Could you check a few things on this drawing? It's one solid part, dimensions in mm from its lowest x, y, z. Give positions to 0.01 mm unless a question says otherwise; leave off trailing zeros. Loops run counter-clockwise (first coordinate to the right, second up) from the corner with the lowest first, then second, coordinate; pieces in that order, holes last.
1. I need wall thicknesses on line 1 along X through (y, z) = (0.45, 4.45); line 2 along Y through (x, z) = (2.6, 4.45); line 3 along Z through (x, y) = (1.4, 1.5). Which ranges of each line are inside material? Lowest first, please.
2. Thinking about a two-plate mould opening in Z: for the marked faces 1, 2 and 3, which applies, +Z half, -Z half, draft (parallel to the pull), parting line (faces both ways), or undercut?
3. Imagine slicing it at D-D (z = 4.25). Count the separate pieces of the cut face and the enclosed holes in it.
4. Imagine slicing it at A-A (y = 1.5). List the corners of the cut face in (x, z) for me.
5. Imagine slicing it at C-C (z = 5.75). List the corners of the cut face in (x, y) for me.
6. For P1, Ø1.3, axis at y = 1.5, z = 4, coming from the +X side; P2, Ø1.5, axis at x = 12.5, z = 1, coming from the +Y side; P3, Ø0.6, axis at x = 6, y = 0.5, coming from the +Z side, each with a flat end and sliding along its axis, tell me the tip position at first contact or that it passes through.
7. Imagine slicing it at B-B (x = 12.25). List the corners of the cut face in (y, z) for me.
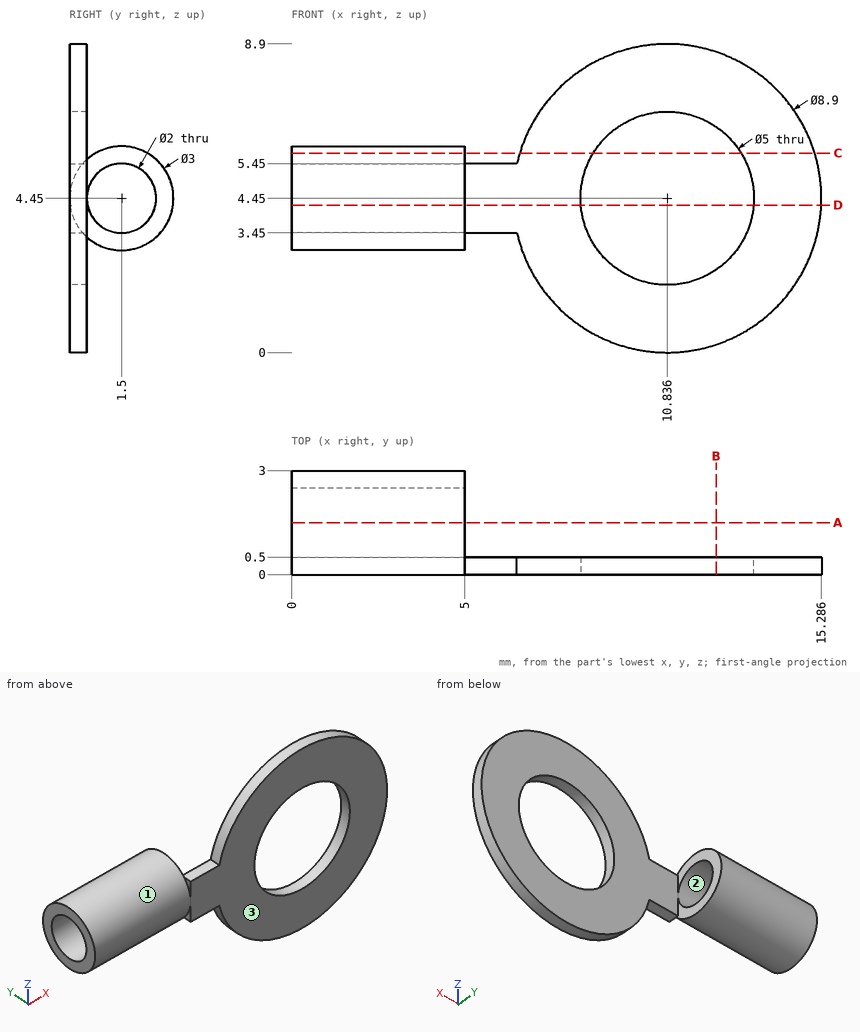
Derived:
1. line 1: x = 0 to 8.34, 13.34 to 15.29
1. line 2: y = 0 to 0.5, 2.5 to 3
1. line 3: z = 2.95 to 3.45, 5.45 to 5.95
2. face 1: parting line
2. face 2: undercut
2. face 3: draft
3. separate pieces: 3
3. enclosed holes: 0
4. outline: (0, 2.95) - (5, 2.95) - (5, 3.45) - (0, 3.45) - close; (0, 5.45) - (5, 5.45) - (5, 5.95) - (0, 5.95) - close
5. outline: (0, 0.75) - (5, 0.75) - (5, 2.25) - (0, 2.25) - close; (6.58, 0) - (8.7, 0) - (8.7, 0.5) - (6.58, 0.5) - close; (12.97, 0) - (15.09, 0) - (15.09, 0.5) - (12.97, 0.5) - close
6. P1: stops at x = 5
6. P2: stops at y = 0.5
6. P3: stops at z = 5.45
7. outline: (0, 0.23) - (0.5, 0.23) - (0.5, 2.39) - (0, 2.39) - close; (0, 6.51) - (0.5, 6.51) - (0.5, 8.67) - (0, 8.67) - close
